from build123d import *

# Parameters (mm, degrees)
F0_W     = 110
F0_H     = 22
F1_DEPTH = 0.8
F2_W     = 3.5
F2_H     = 1
F2_W_2   = 2.5
F2_H_2   = 1.2
F3_DEPTH = 0.801
F4_R     = 0.99999
F2_W_3   = 20
F2_H_3   = 20
F5_DEPTH = 1.35


# Not quite as in the source:
# - a fillet or chamfer is up to 0.001 mm smaller than in the source, because OpenCascade refuses the exact size


with BuildPart() as f1:
    # F0 (on Top) → F1 (new body)
    with BuildSketch(Plane.XY):
        Rectangle(F0_W, F0_H)
    extrude(amount=F1_DEPTH)

    # F2 (on face) → F3 (cut, through all)
    with BuildSketch(Plane.XY.offset(0.8)):
        with BuildLine():
            Line((-55, 1.75), (-55, -1.75))
            ThreePointArc((-55, -1.75), (-53.25, 0), (-55, 1.75))
        make_face()
        with Locations((53.25, 10.5)):
            Rectangle(F2_W, F2_H)
        with Locations((53.25, -10.5)):
            Rectangle(F2_W, F2_H)
        with BuildLine():
            ThreePointArc((52.5, -5.025), (51.9, -5.625), (52.5, -6.225))
            Line((52.5, -6.225), (52.5, -5.025))
        make_face()
        with BuildLine():
            Line((52.5, 5.525), (52.5, 6.725))
            ThreePointArc((52.5, 6.725), (51.9, 6.125), (52.5, 5.525))
        make_face()
        with Locations((53.75, -5.625)):
            Rectangle(F2_W_2, F2_H_2)
        with Locations((53.75, 6.125)):
            Rectangle(F2_W_2, F2_H_2)
    extrude(amount=-F3_DEPTH, mode=Mode.SUBTRACT)

    # F4 (radius 1 in the source; OpenCascade refuses exactly that, so slightly less here)
    f4_edges = [f1.edges().sort_by_distance(p)[0] for p in [
        (51.5, -10, 0.4),
        (51.5, 10, 0.4),
    ]]
    fillet(f4_edges, radius=F4_R)

    # F2 (on face) → F5 (join)
    with BuildSketch(Plane.XY.offset(0.8)):
        with Locations((36.5, 0)):
            Rectangle(F2_W_3, F2_H_3)
        with Locations((11.5, 0)):
            Rectangle(F2_W_3, F2_H_3)
        with Locations((-13.5, 0)):
            Rectangle(F2_W_3, F2_H_3)
        with Locations((-38.5, 0)):
            Rectangle(F2_W_3, F2_H_3)
    extrude(amount=F5_DEPTH)


solid = f1.part
Verification items for the finished model (mm, model axes). Round coordinates to 2 decimals unless told otherwise and drop trailing zeros. Write each loop counter-clockwise with the first axis right and the second up, starting at its lowest first coordinate (ties: lowest second). Pieces come first, ordered by that corner, then holes.
(1) Section check B-B (y = 4). Enter the section's corners in (x, z).
Returned:
outline: (-55, 0) - (55, 0) - (55, 0.8) - (46.5, 0.8) - (46.5, 2.15) - (26.5, 2.15) - (26.5, 0.8) - (21.5, 0.8) - (21.5, 2.15) - (1.5, 2.15) - (1.5, 0.8) - (-3.5, 0.8) - (-3.5, 2.15) - (-23.5, 2.15) - (-23.5, 0.8) - (-28.5, 0.8) - (-28.5, 2.15) - (-48.5, 2.15) - (-48.5, 0.8) - (-55, 0.8) - close
(2) Material ranges on line 1 (X direction, y = 1.75, z = 1.4); line 2 (Y direction, x = 37, z = 1.6); line 3 (Z direction, x = 23, y = -8), recorded low to high.
Returned:
line 1: x = -48.5 to -28.5, -23.5 to -3.5, 1.5 to 21.5, 26.5 to 46.5
line 2: y = -10 to 10
line 3: z = 0 to 0.8
(3) Section check D-D (y = 0). Enter the section's corners in (x, z).
Returned:
outline: (-53.25, 0) - (55, 0) - (55, 0.8) - (46.5, 0.8) - (46.5, 2.15) - (26.5, 2.15) - (26.5, 0.8) - (21.5, 0.8) - (21.5, 2.15) - (1.5, 2.15) - (1.5, 0.8) - (-3.5, 0.8) - (-3.5, 2.15) - (-23.5, 2.15) - (-23.5, 0.8) - (-28.5, 0.8) - (-28.5, 2.15) - (-48.5, 2.15) - (-48.5, 0.8) - (-53.25, 0.8) - close
(4) Section check C-C (x = -2.5). Enter the section's corners in (y, z).
Returned:
outline: (-11, 0) - (11, 0) - (11, 0.8) - (-11, 0.8) - close
(5) Mould release check, pull along Y, two halves, no side actions. Record for faces 1 (the flat face through (-1, 0, 0.8)), 2 (the cylindrical face through (-53.25, -0.04, 0.41)): pulls with the +Y half, pulls with the -Y half, needs draft (parallel to the pull), parting line crosses it, or undercut.
Returned:
face 1: needs draft
face 2: undercut
(6) Depth check by flat-ended pin: pin 1 Ø1.1 at (y, z) = (-2, 1.5) entering from +X; pin 2 Ø0.7 at (x, z) = (15.5, 1.5) entering from +Y; pin 3 Ø0.6 at (x, z) = (54, 0) entering from -Y. Enter the tip coordinate at first touch or a pass-through.
Returned:
pin 1: stops at x = 46.5
pin 2: stops at y = 10
pin 3: stops at y = -10
(7) Section check A-A (z = 1.55). Enter the section's corners in (x, y).
Returned:
outline: (-48.5, -10) - (-28.5, -10) - (-28.5, 10) - (-48.5, 10) - close; (-23.5, -10) - (-3.5, -10) - (-3.5, 10) - (-23.5, 10) - close; (1.5, -10) - (21.5, -10) - (21.5, 10) - (1.5, 10) - close; (26.5, -10) - (46.5, -10) - (46.5, 10) - (26.5, 10) - close
